Study the drawing (mm; zero at the part's minimum x, y, z) and answer. A direction names the side the tool comes from. Coordinates: 2 decimals unless noted, no trailing zeros. Write each loop counter-clockwise with the first axis right and the second up, starting at its lowest first coordinate (ties: lowest second). Pieces come first, ordered by that corner, then holes. Notation, with made-up numbers: (79.25, 55.25) -> (132.25, 55.25) arc R4 ccw to (132.25, 60.25) -> close; hole circle Ø3 at (70, -25). An arc over 180 degrees is marked (long way). Write item = value, one per line. Start each with the question number.
1) Find the intervals of material crossed by line 1 along Z through (x, y) = (4.75, 2); line 2 along Y through (x, z) = (3, 2.8); line 3 along X through (y, z) = (3, 1.2), in increasing order. Write a range as from..to.
2) A tool of negligible diameter and unlimited length cuts with its end or side. For the marked faces 1, 2, 3 and 4, from which of +Z, -Z, +X, -X, +Y, -Y can it reach the whole face along a straight path? Write none if from no direction.
3) Flat-ended cylindrical pins translate along their axes: pin 1 Ø1 at (x, z) = (3.5, 2.5) entering from -Y; pin 2 Ø1.5 at (y, z) = (5.5, 3.5) entering from -X; pin 3 Ø1.2 at (y, z) = (2.5, 2.5) entering from +X; pin 4 Ø0.5 at (x, z) = (3, 3) entering from +Y. Find the tip coordinate at first contact, or state that the pin passes through.
4) Section D-D (y = 2) is taken. Determine the outline of the cut face in (x, z).
5) Section C-C (z = 1.6) is taken. Determine the outline of the cut face in (x, y).
6) Section A-A (y = 3.25) is taken. Determine the outline of the cut face in (x, z).
7) Section B-B (x = 3.25) is taken. Determine the outline of the cut face in (y, z).
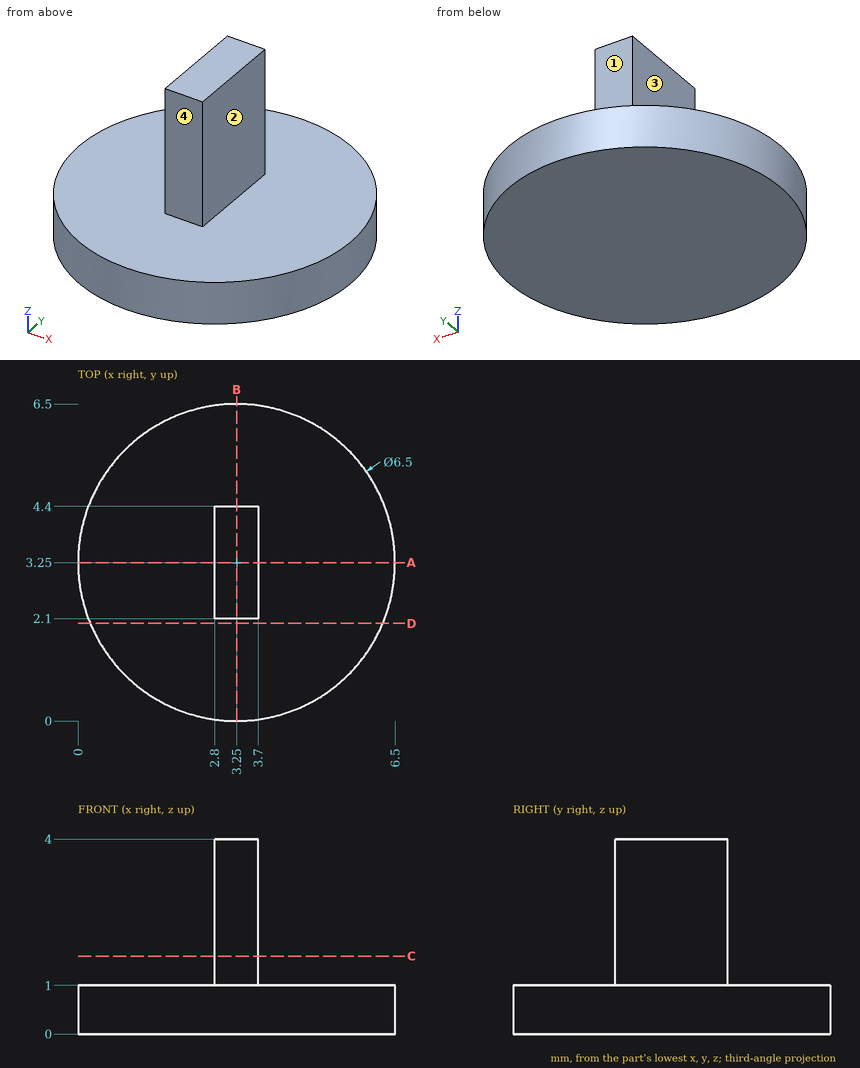
Answer key:
q1.line_1 = 0..1
q1.line_2 = 2.1..4.4
q1.line_3 = 2.8..3.7
q2.face_1 = +Z, +X, -X, +Y
q2.face_2 = +Z, +X, +Y, -Y
q2.face_3 = +Z, -X, +Y, -Y
q2.face_4 = +Z, +X, -X, -Y
q3.pin_1 = 2.1
q3.pin_2 = through
q3.pin_3 = 3.7
q3.pin_4 = 4.4
q4.outline = (0.25, 0) -> (6.25, 0) -> (6.25, 1) -> (0.25, 1) -> close
q5.outline = (2.8, 2.1) -> (3.7, 2.1) -> (3.7, 4.4) -> (2.8, 4.4) -> close
q6.outline = (0, 0) -> (6.5, 0) -> (6.5, 1) -> (3.7, 1) -> (3.7, 4) -> (2.8, 4) -> (2.8, 1) -> (0, 1) -> close
q7.outline = (0, 0) -> (6.5, 0) -> (6.5, 1) -> (4.4, 1) -> (4.4, 4) -> (2.1, 4) -> (2.1, 1) -> (0, 1) -> close
